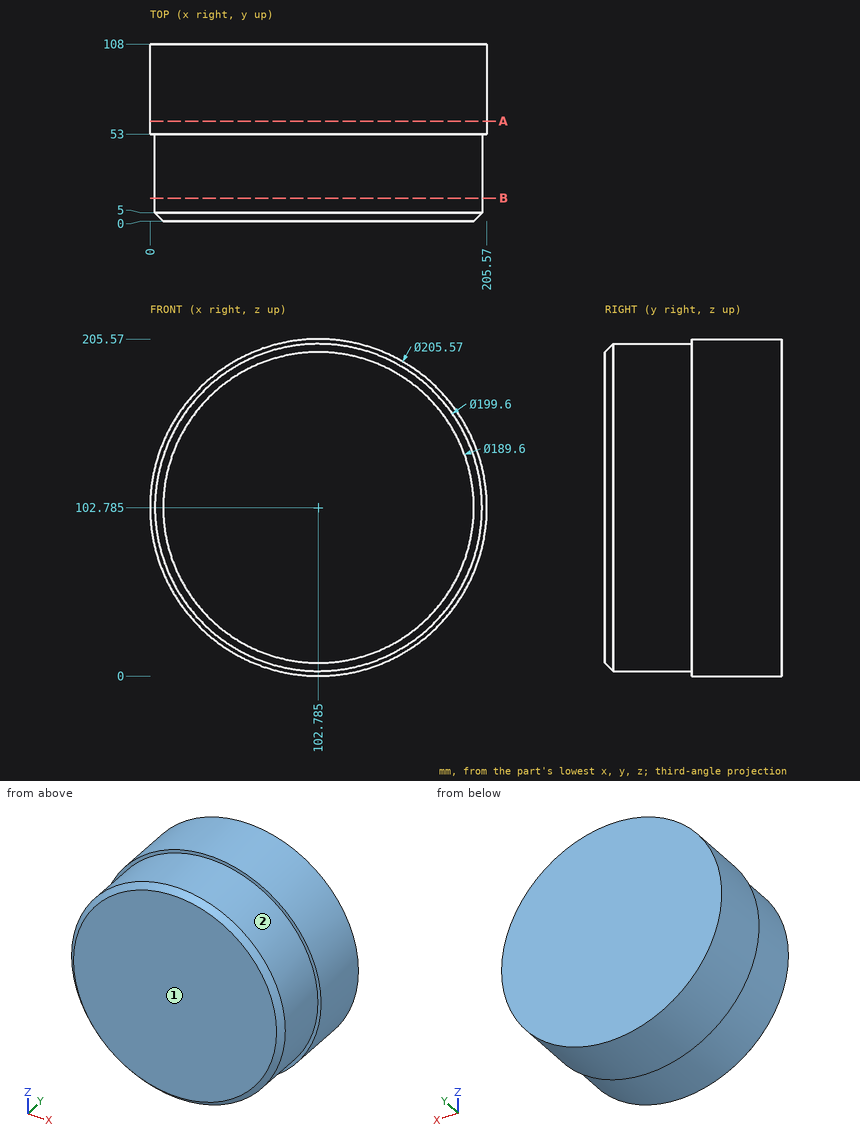
Geometry: see drawing. Coordinates: mm, zero at the bounding-box minimum. A direction names the side the tool comes from. Give positions to 0.01 mm unless a question says otherwise; leave off trailing zeros. Write each loop counter-clockwise with the first axis right and the second up, starting at its lowest first coordinate (ties: lowest second). Pieces come first, ordered by that corner, then holes. Notation, with made-up numbers: (8, 87.5) - (36, 87.5) arc R16 cw to (36, 102.5) - close; hole circle Ø10 at (-24, -38.75). An arc over 180 degrees is marked (long way). Return JSON: item names as keys, results as strings. Group by question number.
1) First-contact query: P1, Ø5, axis at x = 151.5, y = 36.5, coming from the -Z side; P2, Ø1, axis at x = 65, y = 28.5, coming from the -Z side; P3, Ø12, axis at y = 43, z = 98.5, coming from the -X side (3 decimals). Flat tips, straight axial feed; report the tip coordinate or a pass-through.
2) Section B-B on y = 14. Return the cut outline in (x, z) (3 decimals), plus the area to 3 significant figures.
3) Section A-A on y = 61. Return the cut outline in (x, z) (3 decimals), plus the area to 3 significant figures.
4) Line query: line 1 (Y direction, x = 69, z = 194.5); line 2 (X direction, y = 57, z = 102.5); line 3 (Y direction, x = 196.5, z = 71.5). Output: solid intervals per line, ascending.
5) Set-up query: the marked faces 1 and 2. Return all of +Z, -Z, +X, -X, +Y, -Y with unobstructed straight access to the full face (end or side cutting, diameter ignored); none if empty.
Filled in:
{
 "1": {"P1": "stops at z = 14.33", "P2": "stops at z = 10.21", "P3": "stops at x = 2.985"},
 "2": {"outline": "circle Ø199.6 at (102.785, 102.785)", "area": "31,300 mm^2"},
 "3": {"outline": "circle Ø205.57 at (102.785, 102.785)", "area": "33,200 mm^2"},
 "4": {"line 1": "y = 2.94 to 108", "line 2": "x = 0 to 205.57", "line 3": "y = 4 to 108"},
 "5": {"face 1": "+Z, -Z, +X, -X, -Y", "face 2": "-Y"}
}
